from build123d import *

# Parameters (mm, degrees)
F0_R     = 60.481634
F1_DEPTH = 25.4
F2_R     = 27.027248
F3_DEPTH = 76.2
F5_D     = 38.1


with BuildPart() as f1:
    # F0 (on Top) → F1 (new body)
    with BuildSketch(Plane.XY):
        Circle(F0_R)
    extrude(amount=F1_DEPTH)

    # F2 (on face) → F3 (join)
    with BuildSketch(Plane.XY.offset(25.4)):
        Circle(F2_R)
    extrude(amount=F3_DEPTH)

    # F5 (through all)
    with Locations(Plane(origin=(0, 0, 0), x_dir=(1, 0, 0), z_dir=(0, 0, -1))):
        with Locations((0, 0)):
            Hole(F5_D / 2)


solid = f1.part
Check sheet for the modelled part. Datum: model origin and axes. Units: mm. A direction names the side the tool comes from. Coordinates: 2 decimals unless noted, no trailing zeros. Write each loop counter-clockwise with the first axis right and the second up, starting at its lowest first coordinate (ties: lowest second). Pieces come first, ordered by that corner, then holes.
Item 1: Cross-section at A-A on x = 0. Record the boundary of the cut face in (y, z).
Numbers:
outline: (-60.48, 0) - (-19.05, 0) - (-19.05, 101.6) - (-27.03, 101.6) - (-27.03, 25.4) - (-60.48, 25.4) - close; (19.05, 0) - (60.48, 0) - (60.48, 25.4) - (27.03, 25.4) - (27.03, 101.6) - (19.05, 101.6) - close
Item 2: Depth check by flat-ended pin: pin 1 Ø8 at (x, z) = (12.5, 29) entering from +Y; pin 2 Ø6 at (x, z) = (-1.5, 82.5) entering from -Y; pin 3 Ø3 at (x, y) = (-20, 0.5) entering from -Z; pin 4 Ø5 at (x, z) = (-10, 40.5) entering from -Y. Enter the tip coordinate at first touch or a pass-through.
Numbers:
pin 1: stops at y = 59.52
pin 2: stops at y = -27.03
pin 3: stops at z = 0
pin 4: stops at y = -25.97
Item 3: Access from +Z, -Z, +X, -X, +Y, -Y to the whole of each face (thin tool, end or side, straight path). Record for faces 1 (the face through (26, -13, 25.4)), 2 (the face through (5.6, 18.4, 101.6)).
Numbers:
face 1: +Z
face 2: +Z, +X, -X, +Y, -Y
Item 4: Cross-section at D-D on z = 84.5. Record the boundary of the cut face in (x, y).
Numbers:
outline: circle Ø54.05 at (0, 0); hole circle Ø38.1 at (0, 0)
Item 5: Cross-section at C-C on y = -21. Record the boundary of the cut face in (x, z).
Numbers:
outline: (-56.72, 0) - (56.72, 0) - (56.72, 25.4) - (17.01, 25.4) - (17.01, 101.6) - (-17.01, 101.6) - (-17.01, 25.4) - (-56.72, 25.4) - close
Item 6: Mould release check, pull along Y, two halves, no side actions. Record for faces 3 (the face through (12.47, -23.98, 62.97)), 4 (the face through (15.12, 11.59, 51.51)), 5 (the face through (-14, 14, 0)): released by +Y, released by -Y, zero draft, split by the parting line, or undercut.
Numbers:
face 3: split by the parting line
face 4: undercut
face 5: zero draft
Item 7: Scan lines: probe 1 along Y at (x, z) = (0, 24); probe 2 along Y at (x, z) = (0, 38.5); probe 3 along Z at (x, y) = (50.5, 26.5). Record each from-to range of solid material in increasing order.
Numbers:
probe 1: y = -60.48 to -19.05, 19.05 to 60.48
probe 2: y = -27.03 to -19.05, 19.05 to 27.03
probe 3: z = 0 to 25.4
